Autodesk Inventor part; units mm, degrees
ref_plane "YZ Plane" through (0, 0, 0) normal (1, 0, 0) x (0, 1, 0)
ref_plane "XZ Plane" through (0, 0, 0) normal (0, 1, 0) x (-1, 0, 0)
ref_plane "XY Plane" through (0, 0, 0) normal (0, 0, 1) x (1, 0, 0)
sketch "Sketch1" plane through (0, 0, 0) normal (0, 0, 1) x (1, 0, 0)
  line L0 (0, 17.6499) -> (25.7669, 17.6499)
  line L1 (25.7669, 17.6499) -> (25.7669, 0)
  line L2 (25.7669, 0) -> (0, 0)
  line L3 (0, 0) -> (0, 17.6499)
  line L4 (25.7669, 17.6499) -> (0, 17.6499)
  line L5 (0, 17.6499) -> (0, 16.3405)
  line L6 (0, 16.3405) -> (25.7669, 16.3405)
  line L7 (25.7669, 16.3405) -> (25.7669, 17.6499)
  line L8 (25.7669, 0) -> (0, 0)
  line L9 (0, 0) -> (0, 1.306)
  line L10 (0, 1.306) -> (25.7669, 1.306)
  line L11 (25.7669, 1.306) -> (25.7669, 0)
  dimension "d0" = 17.65
  dimension "d1" = 15.0345
  dimension "d2" = 1.3094
  dimension "d3" = 1.306
  dimension "d4" = 25.7669
extrude "Extrusion1" add sketch "Sketch1" along normal blind 1.5
extrude "Extrusion2" add sketch "Sketch1" against normal blind 9.3 contours L0 L1 L6 L3 | L10 L1 L2 L3
properties part number "Cover"
Geometry check sheet. Reference: the model listing, model coordinates, mm. A direction names the side the tool comes from. Coordinates: 2 decimals unless noted, no trailing zeros. Order: outer loops, then holes, each group sorted by start corner. A loop starts at its lowest first (then second) coordinate and runs counter-clockwise, first axis right, second up.
Item 1: Mould release check, pull along Y, two halves, no side actions. Record for faces 3 (the flat face through (13, 17.65, -4)), 4 (the flat face through (13, 1.306, -5)), 5 (the flat face through (13, 9, 0)), 6 (the flat face through (13, 9, 1.5)): released by +Y, released by -Y, zero draft, split by the parting line, or undercut.
Item 2: Section check C-C (y = 15). Enter the section's corners in (x, z).
Item 3: Section check A-A (z = -2). Enter the section's corners in (x, y), plus the area to 3 significant figures.
Item 4: Section check B-B (x = 9). Enter the section's corners in (y, z).
Item 5: Scan lines: line 1 along Y through (x, z) = (6, -2.25); line 2 along Z through (x, y) = (6, 13.5). Record each from-to range of solid material in increasing order.
Item 6: Depth check by flat-ended pin: pin 1 (4.5 mm diameter, centred on x = 10, y = 5.5, fed in from -Z). Enter the tip coordinate at first touch or a pass-through.
Item 7: Tool access check on faces 1 (the flat face through (25.767, 8.9, 0.5)), 2 (the flat face through (13, 16.34, -5)). Record the directions out of +Z, -Z, +X, -X, +Y, -Y that give a thin tool (end or side, any length) a straight path to the whole face; none if there is none.
Check sheet entries:
1. face 3: released by +Y
1. face 4: undercut
1. face 5: undercut
1. face 6: zero draft
2. outline: (0, 0) - (25.77, 0) - (25.77, 1.5) - (0, 1.5) - close
3. outline: (0, 0) - (25.77, 0) - (25.77, 1.31) - (0, 1.31) - close; (0, 16.34) - (25.77, 16.34) - (25.77, 17.65) - (0, 17.65) - close
3. area: 67.4 mm2
4. outline: (0, -9.3) - (1.31, -9.3) - (1.31, 0) - (16.34, 0) - (16.34, -9.3) - (17.65, -9.3) - (17.65, 1.5) - (0, 1.5) - close
5. line 1: y = 0 to 1.31, 16.34 to 17.65
5. line 2: z = 0 to 1.5
6. pin 1: stops at z = 0
7. face 1: +Z, -Z, +X, +Y, -Y
7. face 2: -Z, +X, -X
